Verification items for this drawing (mm, ordinates from the low corner). A direction names the side the tool comes from. Coordinates: 2 decimals unless noted, no trailing zeros. Write each loop counter-clockwise with the first axis right and the second up, starting at its lowest first coordinate (ties: lowest second). Pieces come first, ordered by that corner, then holes. Notation, with made-up numbers: (-6, -9) -> (45, -9) arc R10 cw to (45, -4) -> close; hole circle Ø8 at (53, -24.5). An arc over 180 degrees is marked (long way). Use CSV: the item, a comma, the result in double quotes.
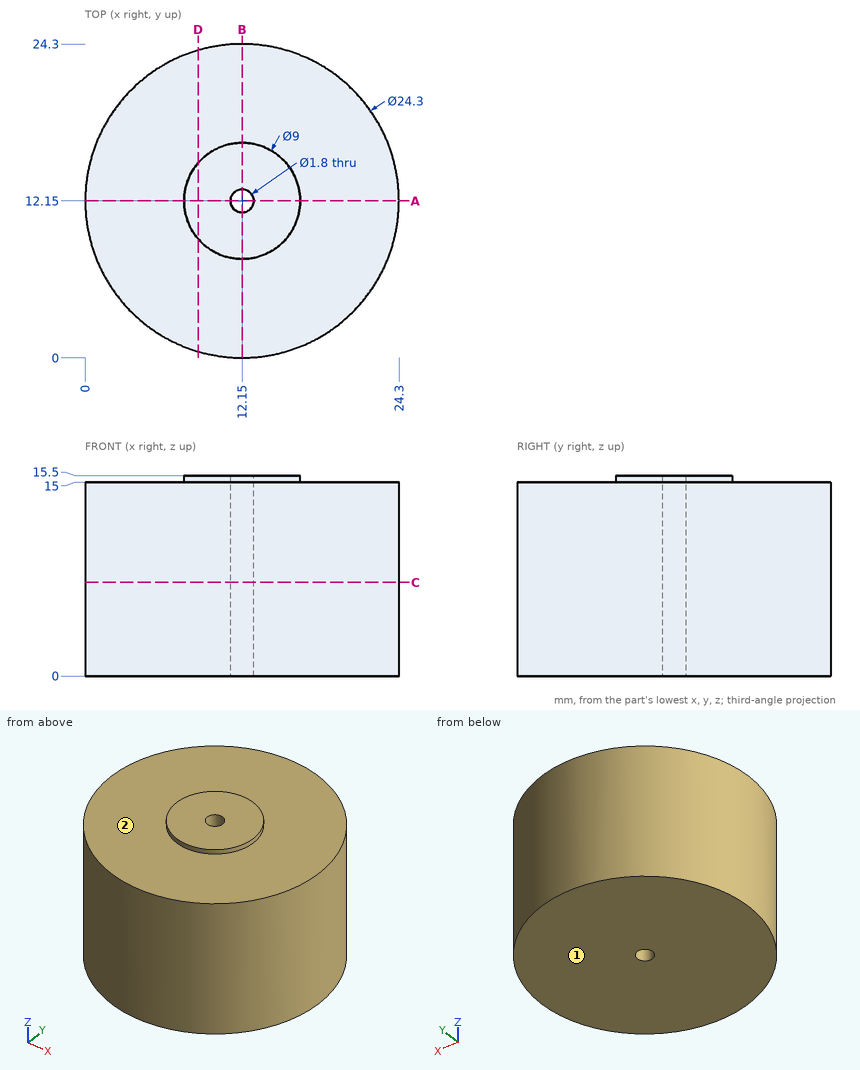
1) Set-up check for the marked faces 1 and 2: record each of +Z, -Z, +X, -X, +Y, -Y from which the full face is reachable in a straight line by a thin tool's end or side.
Return value:
face 1,"-Z, +X, -X, +Y, -Y"
face 2,"+Z"
2) Cross-section at A-A (y = 12.15). Record the boundary of the cut face in (x, z), plus the area to 3 significant figures.
Return value:
outline,"(0, 0) -> (11.25, 0) -> (11.25, 15.5) -> (7.65, 15.5) -> (7.65, 15) -> (0, 15) -> close; (13.05, 0) -> (24.3, 0) -> (24.3, 15) -> (16.65, 15) -> (16.65, 15.5) -> (13.05, 15.5) -> close"
area,"341 mm2"
3) Scan lines: L1, parallel to Y at x = 12.15, z = 7.5; L2, parallel to Z at x = 7.5, y = 9; L3, parallel to X at y = 12, z = 8. Record each from-to range of solid material in increasing order.
Return value:
L1,"0 to 11.25, 13.05 to 24.3"
L2,"0 to 15"
L3,"0 to 11.26, 13.04 to 24.3"
4) Cross-section at C-C (z = 7.25). Record the boundary of the cut face in (x, y).
Return value:
outline,"circle Ø24.3 at (12.15, 12.15); hole circle Ø1.8 at (12.15, 12.15)"
5) Gauge pin test, flat ends, axial feed: pin 1 (3 mm diameter, centred on x = 19, z = 12, fed in from +Y); pin 2 (8 mm diameter, centred on y = 2.5, z = 12.5, fed in from +X); pin 3 (5 mm diameter, centred on x = 19, y = 16.5, fed in from +Z). Record the tip position at first contact, or that the pin passes through.
Return value:
pin 1,"y = 23.06"
pin 2,"x = 22.91"
pin 3,"z = 15"
6) Cross-section at D-D (x = 8.75). Record the boundary of the cut face in (y, z).
Return value:
outline,"(0.49, 0) -> (23.81, 0) -> (23.81, 15) -> (15.1, 15) -> (15.1, 15.5) -> (9.2, 15.5) -> (9.2, 15) -> (0.49, 15) -> close"
